```python
from build123d import *

# Parameters (mm, degrees)
SM_BASE_FLANGE_1_DEPTH           = 30
SKETCH_5_R                       = 3
CUT_EXTRUDE_3_DEPTH              = 10
SM_EDGE_FLANGE_1_STRIP_W         = 6.2
SM_EDGE_FLANGE_1_STRIP_H         = 1
SM_EDGE_FLANGE_1_STRIP_CUT_DEPTH = 30
SM_EDGE_FLANGE_1_DEPTH           = 30
CHAMFER_1_SIZE                   = 10
SKETCH_10_R                      = 4.25
CUT_EXTRUDE_4_DEPTH              = 10
CHAMFER_2_SIZE                   = 5


# Sheet-metal steps are written as plain solids
with BuildPart() as part:
    # Sketch 1 → Базовая кромка1 (new body)
    with BuildSketch(Plane.XY):
        with BuildLine():
            Line((0, 12), (0, 1.1))
            ThreePointArc((0, 1.1), (0.322182541, 0.322182541), (1.1, 0))
            Line((1.1, 0), (13, 0))
            Line((13, 0), (13, -1))
            Line((13, -1), (1.1, -1))
            ThreePointArc((1.1, -1), (-0.38492424, -0.38492424), (-1, 1.1))
            Line((-1, 1.1), (-1, 12))
            Line((-1, 12), (0, 12))
        make_face()
    extrude(amount=SM_BASE_FLANGE_1_DEPTH)

    # Эскиз5 → Вырез-Вытянуть3 (cut)
    with BuildSketch(Plane(origin=(0, 0, 0), x_dir=(1, 0, 0), z_dir=(0, 1, 0))):
        with Locations(Location((7, -17.618648825, 0), (0, 0, 270))):
            Circle(SKETCH_5_R)
    extrude(amount=-CUT_EXTRUDE_3_DEPTH, mode=Mode.SUBTRACT)

    # Ребро-кромка1 strip (across the edge) → Ребро-кромка1 strip cut (cut)
    with BuildSketch(Plane(origin=(-1, 12, 30), x_dir=(0, -1, 0), z_dir=(0, 0, -1))):
        with Locations((-1, -0.5)):
            Rectangle(SM_EDGE_FLANGE_1_STRIP_W, SM_EDGE_FLANGE_1_STRIP_H)
    extrude(amount=SM_EDGE_FLANGE_1_STRIP_CUT_DEPTH, mode=Mode.SUBTRACT)

    # Ребро-кромка1 section (across the edge) → Ребро-кромка1 (add)
    with BuildSketch(Plane(origin=(-1, 12, 30), x_dir=(0, -1, 0), z_dir=(0, 0, -1))):
        with BuildLine():
            Line((0, 1.1), (0, 15))
            Line((0, 15), (1, 15))
            Line((1, 15), (1, 1.1))
            ThreePointArc((1, 1.1), (1.322182541, 0.322182541), (2.1, 0))
            Line((2.1, 0), (2.1, -1))
            ThreePointArc((2.1, -1), (0.61507576, -0.38492424), (0, 1.1))
        make_face()
    extrude(amount=SM_EDGE_FLANGE_1_DEPTH)

    # Фаска1
    chamfer_1_edges = [part.edges().sort_by_distance(p)[0] for p in [
        (-16, 11.5, 30),
        (-16, 11.5, 0),
    ]]
    chamfer(chamfer_1_edges, length=CHAMFER_1_SIZE)

    # Эскиз10 → Вырез-Вытянуть4 (cut)
    with BuildSketch(Plane(origin=(0, 12, 0), x_dir=(1, 0, 0), z_dir=(0, 1, 0))):
        with Locations(Location((-11.054624514, -15, 0), (0, 0, 180))):
            Circle(SKETCH_10_R)
    extrude(amount=-CUT_EXTRUDE_4_DEPTH, mode=Mode.SUBTRACT)

    # Фаска2
    chamfer_2_edges = [part.edges().sort_by_distance(p)[0] for p in [
        (13, -0.5, 30),
        (13, -0.5, 0),
    ]]
    chamfer(chamfer_2_edges, length=CHAMFER_2_SIZE)


solid = part.part
```
Input: part model. Units: mm. Frame: model coordinates. A direction names the side the tool comes from. Coordinates: 2 decimals unless noted, no trailing zeros. Write each loop counter-clockwise with the first axis right and the second up, starting at its lowest first coordinate (ties: lowest second). Pieces come first, ordered by that corner, then holes. Notation, with made-up numbers: (50.25, 70.5) - (109.25, 70.5) arc R20 ccw to (109.25, 93.5) - close; hole circle Ø1 at (-40, 71). An arc over 180 degrees is marked (long way). Put each result on its own line as item: value. Start each with the question number.
1) Mould query, pull axis X, two halves, no side actions, for faces 4 (the face through (8.5, -1, 14.8)), 5 (the face through (-16, 11.5, 15.1)), 6 (the face through (4.07, -0.49, 16.97)). Classes: pulls with the +X half, pulls with the -X half, needs draft (parallel to the pull), parting line crosses it, or undercut.
2) Ray query, L1, parallel to X at y = 8.5, z = 24; L2, parallel to Y at x = -3.5, z = 20. Return the intervals inside material, ascending.
3) Cut plane C-C (z = 7). Return the cut outline in (x, y).
4) Reachability of faces 1 (the face through (-1, 5, 15)), 2 (the face through (0, 6, 15)), 3 (the face through (-0.6, 5, 30)) from +Z, -Z, +X, -X, +Y, -Y: full face, straight path, thin tool, end or side. Return the list, or none.
5) Cut plane A-A (x = 7). Return the cut outline in (y, z), plus the area to 3 significant figures.
6) Cut plane B-B (z = 14). Return the cut outline in (x, y), plus the area to 3 significant figures.
7) Contact query for flat-ended pins moving along their axis: pin 1 (6 mm diameter, centred on y = 7.5, z = 10, fed in from -X); pin 2 (1.5 mm diameter, centred on y = 8, z = 7, fed in from +X); pin 3 (1 mm diameter, centred on x = 4.5, y = 2, fed in from +Z); pin 4 (4 mm diameter, centred on x = -7.5, z = 20, fed in from -Y). Output: stop coordinate, or through.
8) Cut plane D-D (y = 2.25). Return the cut outline in (x, z), plus the area to 3 significant figures.
Resolved:
1. face 4: needs draft
1. face 5: pulls with the -X half
1. face 6: undercut
2. L1: x = -1 to 0
2. L2: y = 11 to 12
3. outline: (-13, 11) - (-2.1, 11) arc R1.1 cw to (-1, 9.9) - (-1, 1.1) arc R2.1 ccw to (1.1, -1) - (13, -1) - (13, 0) - (1.1, 0) arc R1.1 cw to (0, 1.1) - (0, 9.9) arc R2.1 ccw to (-2.1, 12) - (-13, 12) - close
4. face 1: +Z, -Z, -X, -Y
4. face 2: +Z, -Z, +X, +Y
4. face 3: +Z, +X, -X, +Y, -Y
5. outline: (-1, 0) - (0, 0) - (0, 14.62) - (-1, 14.62) - close; (-1, 20.62) - (0, 20.62) - (0, 30) - (-1, 30) - close
5. area: 24.0 mm2
6. outline: (-16, 11) - (-15.19, 11) - (-15.19, 12) - (-16, 12) - close; (-6.92, 11) - (-2.1, 11) arc R1.1 cw to (-1, 9.9) - (-1, 1.1) arc R2.1 ccw to (1.1, -1) - (13, -1) - (13, 0) - (1.1, 0) arc R1.1 cw to (0, 1.1) - (0, 9.9) arc R2.1 ccw to (-2.1, 12) - (-6.92, 12) - close
6. area: 31.4 mm2
7. pin 1: stops at x = -1.18
7. pin 2: stops at x = 0
7. pin 3: passes through
7. pin 4: stops at y = 11
8. outline: (-1, 0) - (0, 0) - (0, 30) - (-1, 30) - close
8. area: 30.0 mm2
